Geometry check sheet. Reference: drawing and pictorial views, mm from the part's lowest x, y, z. Round coordinates to 2 decimals unless told otherwise and drop trailing zeros. Order: outer loops, then holes, each group sorted by start corner. A loop starts at its lowest first (then second) coordinate and runs counter-clockwise, first axis right, second up. Notation, with made-up numbers: (9, 71) -> (27, 71) arc R17 cw to (27, 96) -> close; hole circle Ø5 at (43, 74). An arc over 180 degrees is marked (long way). Put each result on its own line as item: value.
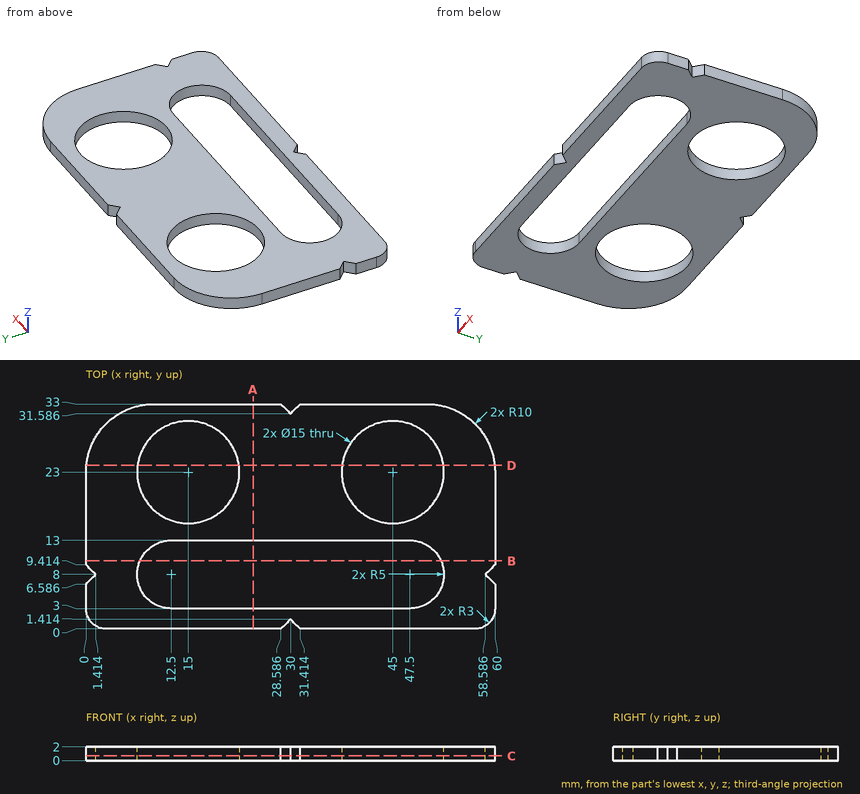
Item 1: Sectioned sample at B-B, the plane y = 10. Record the boundary of the cut face in (x, z), then the cut area to 3 significant figures.
Geometry check:
outline: (0, 0) -> (7.92, 0) -> (7.92, 2) -> (0, 2) -> close; (52.08, 0) -> (60, 0) -> (60, 2) -> (52.08, 2) -> close
area: 31.7 mm2
Item 2: Sectioned sample at A-A, the plane x = 24.5. Record the boundary of the cut face in (y, z).
Geometry check:
outline: (0, 0) -> (3, 0) -> (3, 2) -> (0, 2) -> close; (13, 0) -> (33, 0) -> (33, 2) -> (13, 2) -> close
Item 3: Material ranges on line 1 along Y through (x, z) = (15, 1.1); line 2 along Y through (x, z) = (25, 1.35); line 3 along Y through (x, z) = (46.5, 0.2), recorded low to high.
Geometry check:
line 1: 0 to 3, 13 to 15.5, 30.5 to 33
line 2: 0 to 3, 13 to 33
line 3: 0 to 3, 13 to 15.65, 30.35 to 33
Item 4: Sectioned sample at C-C, the plane z = 0.7. Record the boundary of the cut face in (x, y), then the cut area to 3 significant figures.
Geometry check:
outline: (0, 3) arc R3 ccw to (3, 0) -> (28.59, 0) -> (30, 1.41) -> (31.41, 0) -> (57, 0) arc R3 ccw to (60, 3) -> (60, 6.59) -> (58.59, 8) -> (60, 9.41) -> (60, 23) arc R10 ccw to (50, 33) -> (31.41, 33) -> (30, 31.59) -> (28.59, 33) -> (10, 33) arc R10 ccw to (0, 23) -> (0, 9.41) -> (1.41, 8) -> (0, 6.59) -> close; hole circle Ø15 at (15, 23); hole (12.5, 3) -> (47.5, 3) arc R5 ccw to (47.5, 13) -> (12.5, 13) arc R5 ccw to start; hole circle Ø15 at (45, 23)
area: 1,140 mm2
Item 5: Sectioned sample at D-D, the plane y = 24. Record the boundary of the cut face in (x, z).
Geometry check:
outline: (0.05, 0) -> (7.57, 0) -> (7.57, 2) -> (0.05, 2) -> close; (22.43, 0) -> (37.57, 0) -> (37.57, 2) -> (22.43, 2) -> close; (52.43, 0) -> (59.95, 0) -> (59.95, 2) -> (52.43, 2) -> close
Item 6: Depth check by flat-ended pin: pin 1 Ø12 at (x, y) = (45, 23) entering from -Z; pin 2 Ø2 at (x, y) = (36, 20) entering from -Z. Enter the tip coordinate at first touch or a pass-through.
Geometry check:
pin 1: through
pin 2: z = 0
